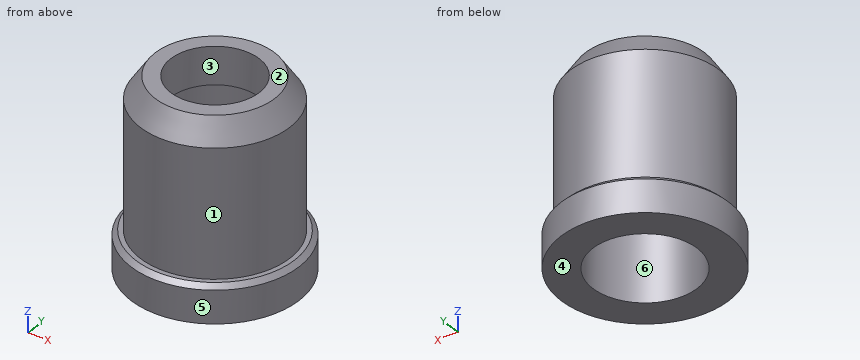
from build123d import *

# Parameters (mm, degrees)
F2_SIZE2 = 3.81
F2_SIZE  = 2.54
F3_SIZE  = 0.7874


with BuildPart() as f1:
    # F0 (on Front) → F1 (revolve)
    with BuildSketch(Plane.XZ):
        Polygon((-14.2875, 0), (-8.89, 0), (-8.89, 25.4), (-7.5311, 25.4), (-7.5311, 31.75), (-12.7, 31.75), (-12.7, 6.35), (-14.2875, 6.35), align=None)
    revolve(axis=Axis((0, 0, 7.331744), (0, 0, -1)))

    # F2
    f2_edges = [f1.edges().sort_by_distance(p)[0] for p in [
        (12.7, 0, 31.75),
    ]]
    chamfer(f2_edges, length=F2_SIZE, length2=F2_SIZE2)

    # F3
    f3_edges = [f1.edges().sort_by_distance(p)[0] for p in [
        (14.2875, 0, 6.35),
    ]]
    chamfer(f3_edges, length=F3_SIZE)


solid = f1.part
Source: CAD feature listing. Evaluate the final solid. Frame: model axes, mm. Face numbers are marked on the shaded views. A direction names the side the tool comes from. Round coordinates to 2 decimals unless told otherwise and drop trailing zeros. Write each loop counter-clockwise with the first axis right and the second up, starting at its lowest first coordinate (ties: lowest second). Pieces come first, ordered by that corner, then holes. Notation, with made-up numbers: (53, 23.25) - (72, 23.25) arc R24 ccw to (72, 51.25) - close; hole circle Ø11 at (76.25, -35.75). An arc over 180 degrees is marked (long way). Use CSV: the item, a comma, the result in double quotes. Start each with the question number.
(1) Cut plane C-C, the plane z = 27. Return loops of the section in (x, y), and give its area (3 significant figures).
(2) First-contact query: pin 1 Ø1.5 at (x, z) = (-8, 26.5) entering from +Y; pin 2 Ø12 at (y, z) = (3.5, 26) entering from -X; pin 3 Ø1.5 at (x, z) = (-6.5, 9.5) entering from -Y. Flat tips, straight axial feed; report the tip coordinate or a pass-through.
(3) Set-up query: the marked faces 1 and 2. Return all of +Z, -Z, +X, -X, +Y, -Y with unobstructed straight access to the full face (end or side cutting, diameter ignored); none if empty.
(4) Material intervals for probe 1 along Y at (x, z) = (0, 27.5); probe 2 along Y at (x, z) = (0, 8.5); probe 3 along Z at (x, y) = (-12.25, 5.5), sorted ascending. Write a range as [from, to].
(5) Mould query, pull axis X, two halves, no side actions, for the marked faces 3, 4, 5 and 6. Classes: pulls with the +X half, pulls with the -X half, needs draft (parallel to the pull), parting line crosses it, or undercut.
(6) Cut plane A-A, the plane y = 0. Return loops of the section in (x, z), and give its area (3 significant figures).
Geometry says:
1,outline,"circle Ø25.4 at (0, 0); hole circle Ø15.06 at (0, 0)"
1,area,"329 mm²"
2,pin 1,"y = 10.43"
2,pin 2,"x = -12.7"
2,pin 3,"y = -11.32"
3,face 1,"+Z"
3,face 2,"+Z, +X, -X, +Y, -Y"
4,probe 1,"[-12.7, -7.53], [7.53, 12.7]"
4,probe 2,"[-12.7, -8.89], [8.89, 12.7]"
4,probe 3,"[0, 6.35]"
5,face 3,"undercut"
5,face 4,"needs draft"
5,face 5,"parting line crosses it"
5,face 6,"undercut"
6,outline,"(-14.29, 0) - (-8.89, 0) - (-8.89, 25.4) - (-7.53, 25.4) - (-7.53, 31.75) - (-10.16, 31.75) - (-12.7, 27.94) - (-12.7, 6.35) - (-13.5, 6.35) - (-14.29, 5.56) - close; (7.53, 25.4) - (8.89, 25.4) - (8.89, 0) - (14.29, 0) - (14.29, 5.56) - (13.5, 6.35) - (12.7, 6.35) - (12.7, 27.94) - (10.16, 31.75) - (7.53, 31.75) - close"
6,area,"269 mm²"
